```python
from build123d import *

# Parameters (mm, degrees)
BOSS_EXTRUDE1_DEPTH = 44.45
FILLET1_R           = 6.35
SHELL1_T            = -1.5875
CUT_EXTRUDE1_REACH  = 132.02
SKETCH2_R           = 2.7051


with BuildPart() as part:
    # Sketch1 → Boss-Extrude1 (new body)
    with BuildSketch(Plane.XY):
        with BuildLine():
            Line((-103.1748, 50.8), (103.1748, 50.8))
            ThreePointArc((103.1748, 50.8), (108.796440332, 48.471440332), (111.125, 42.8498))
            Line((111.125, 42.8498), (111.125, -42.8498))
            ThreePointArc((111.125, -42.8498), (108.796440332, -48.471440332), (103.1748, -50.8))
            Line((103.1748, -50.8), (-103.1748, -50.8))
            ThreePointArc((-103.1748, -50.8), (-108.796440332, -48.471440332), (-111.125, -42.8498))
            Line((-111.125, -42.8498), (-111.125, 42.8498))
            ThreePointArc((-111.125, 42.8498), (-108.796440332, 48.471440332), (-103.1748, 50.8))
        make_face()
    extrude(amount=BOSS_EXTRUDE1_DEPTH)

    # Fillet1
    fillet1_edges = [part.edges().sort_by_distance(p)[0] for p in [
        (108.796440332, -48.471440332, 44.45),
        (111.125, 0, 44.45),
        (108.796440332, 48.471440332, 44.45),
        (0, 50.8, 44.45),
        (-108.796440332, 48.471440332, 44.45),
        (-111.125, 0, 44.45),
        (-108.796440332, -48.471440332, 44.45),
        (0, -50.8, 44.45),
    ]]
    fillet(fillet1_edges, radius=FILLET1_R)

    # Shell1
    shell1_openings = [part.faces().sort_by_distance(p)[0] for p in [
        (0, 0, 0),
    ]]
    offset(amount=SHELL1_T, openings=shell1_openings, kind=Kind.INTERSECTION)

    # Sketch2 → Cut-Extrude1 (cut, up to next)
    with BuildSketch(Plane.XY.offset(44.45), mode=Mode.PRIVATE) as cut_extrude1_sk1:
        with Locations((0, 39.6875)):
            Circle(SKETCH2_R)
    cut_extrude1_tool1 = extrude(cut_extrude1_sk1.sketch, amount=-CUT_EXTRUDE1_REACH, mode=Mode.PRIVATE) & part.part
    # Sketch2 → Cut-Extrude1 (cut, up to next)
    with BuildSketch(Plane.XY.offset(44.45), mode=Mode.PRIVATE) as cut_extrude1_sk2:
        with Locations((0, -39.6875)):
            Circle(SKETCH2_R)
    cut_extrude1_tool2 = extrude(cut_extrude1_sk2.sketch, amount=-CUT_EXTRUDE1_REACH, mode=Mode.PRIVATE) & part.part
    # Sketch2 → Cut-Extrude1 (cut, up to next)
    with BuildSketch(Plane.XY.offset(44.45), mode=Mode.PRIVATE) as cut_extrude1_sk3:
        with Locations((100.0125, 0)):
            Circle(SKETCH2_R)
    cut_extrude1_tool3 = extrude(cut_extrude1_sk3.sketch, amount=-CUT_EXTRUDE1_REACH, mode=Mode.PRIVATE) & part.part
    # Sketch2 → Cut-Extrude1 (cut, up to next)
    with BuildSketch(Plane.XY.offset(44.45), mode=Mode.PRIVATE) as cut_extrude1_sk4:
        with Locations((-100.0125, 0)):
            Circle(SKETCH2_R)
    cut_extrude1_tool4 = extrude(cut_extrude1_sk4.sketch, amount=-CUT_EXTRUDE1_REACH, mode=Mode.PRIVATE) & part.part
    add(cut_extrude1_tool1.solids().sort_by_distance((0, 39.6875, 44.45))[0], mode=Mode.SUBTRACT)
    add(cut_extrude1_tool2.solids().sort_by_distance((0, -39.6875, 44.45))[0], mode=Mode.SUBTRACT)
    add(cut_extrude1_tool3.solids().sort_by_distance((100.0125, 0, 44.45))[0], mode=Mode.SUBTRACT)
    add(cut_extrude1_tool4.solids().sort_by_distance((-100.0125, 0, 44.45))[0], mode=Mode.SUBTRACT)


solid = part.part
```
Check sheet for the modelled part. Datum: model origin and axes. Units: mm. A direction names the side the tool comes from. Coordinates: 2 decimals unless noted, no trailing zeros. Order: outer loops, then holes, each group sorted by start corner. A loop starts at its lowest first (then second) coordinate and runs counter-clockwise, first axis right, second up. Notation, with made-up numbers: M -21,44.25 L 20,44.25 A24 cw 20,67.25 Z; hole C -27.75,52.25 d3. An arc over 180 degrees is marked long. Write each question's results on one line, items separated by ' | '. Start each with the question number.
1. Access from +Z, -Z, +X, -X, +Y, -Y to the whole of each face (thin tool, end or side, straight path). Record for faces 1 (the face through (108, 47, 19)), 2 (the face through (1.454, -37.407, 43.667)).
2. Mould release check, pull along X, two halves, no side actions. Record for faces 3 (the face through (108.734, 48.533, 18.783)), 4 (the face through (-108.734, -48.533, 18.783)), 5 (the face through (1.45, 41.97, 43.67)): +X half, -X half, draft (parallel to the pull), parting line (faces both ways), or undercut.
3. Cross-section at A-A on x = 0. State how many separate pieces and enclosed holes the cut face has, and give its area (3 significant figures).
4. Material ranges on probe 1 along X at (y, z) = (-15, 19) (1 decimal); probe 2 along Y at (x, z) = (-50, 26); probe 3 along Y at (x, z) = (0, 43.8), recorded low to high.
5. Cross-section at C-C on z = 36. Record the cut outline in (x, y) (1 decimal), and give its area (3 significant figures).
6. Go/stop test with a flat-tipped pin: P1, Ø10, axis at x = -66, y = 0, coming from the -Z side. Record where the tip stops, or that it passes through.
Checks:
1) face 1: -Z | face 2: +Z, -Z
2) face 3: +X half | face 4: -X half | face 5: undercut
3) separate pieces: 3 | enclosed holes: 0 | area: 273 mm²
4) probe 1: x = -111.1 to -109.5, 109.5 to 111.1 | probe 2: y = -50.8 to -49.21, 49.21 to 50.8 | probe 3: y = -47.25 to -42.39, -36.98 to 36.98, 42.39 to 47.25
5) outline: M -111.1,-42.8 A8 ccw -103.2,-50.8 L 103.2,-50.8 A8 ccw 111.1,-42.8 L 111.1,42.8 A8 ccw 103.2,50.8 L -103.2,50.8 A8 ccw -111.1,42.8 Z; hole M -109.5,-42.8 A6.4 ccw -103.2,-49.2 L 103.2,-49.2 A6.4 ccw 109.5,-42.8 L 109.5,42.8 A6.4 ccw 103.2,49.2 L -103.2,49.2 A6.4 ccw -109.5,42.8 Z | area: 999 mm²
6) P1: stops at z = 42.86
